from build123d import *

# Parameters (mm, degrees)
F1_DEPTH = 25
F2_R     = 1.5
F3_DEPTH = 25
F4_W     = 10
F4_H     = 10
F4_R     = 1.5
F5_DEPTH = 5
F6_SIZE  = 1
F7_SIZE  = 1


with BuildPart() as f1:
    # F0 (on Front) → F1 (new body)
    with BuildSketch(Plane.XZ):
        Polygon((0, -3.6), (0, 3.6), (10, 3.6), (10, 6.1), (-2.5, 6.1), (-2.5, -6.1), (15, -6.1), (15, -3.6), align=None)
    extrude(amount=F1_DEPTH)

    # F2 (on face) → F3 (cut)
    with BuildSketch(Plane.XY.offset(6.1)):
        with Locations((5.5, -5.5)):
            Circle(F2_R)
    extrude(amount=-F3_DEPTH, mode=Mode.SUBTRACT)

    # F4 (on face) → F5 (cut)
    with BuildSketch(Plane.XY.offset(6.1)):
        with Locations((5, -5)):
            Rectangle(F4_W, F4_H)
        with Locations((5.5, -5.5)):
            Circle(F4_R, mode=Mode.SUBTRACT)
    extrude(amount=-F5_DEPTH, mode=Mode.SUBTRACT)

    # F6
    f6_edges = [f1.edges().sort_by_distance(p)[0] for p in [
        (-2.5, -12.5, 6.1),
        (-2.5, -12.5, -6.1),
        (15, -12.5, -6.1),
        (6.25, -25, -6.1),
        (6.25, 0, -6.1),
        (-2.5, 0, 0),
    ]]
    chamfer(f6_edges, length=F6_SIZE)

    # F7
    f7_edges = [f1.edges().sort_by_distance(p)[0] for p in [
        (-0.75, 0, 6.1),
    ]]
    chamfer(f7_edges, length=F7_SIZE)


solid = f1.part
Check sheet for the modelled part. Datum: model origin and axes. Units: mm. A direction names the side the tool comes from. Coordinates: 2 decimals unless noted, no trailing zeros. Loops run counter-clockwise (first coordinate to the right, second up) from the corner with the lowest first, then second, coordinate; pieces in that order, holes last. Notation, with made-up numbers: (6.25, -30.5) -> (21.25, -30.5) arc R5 ccw to (21.25, -23.5) -> close; hole circle Ø9 at (49, 16.5). An arc over 180 degrees is marked (long way). Write item = value, one per line. Start each with the question number.
1. Section check D-D on z = -3. Record the cut outline in (x, y), then the cut area to 3 significant figures.
2. Material ranges on line 1 (Y direction, x = 5.5, z = -4.15); line 2 (Z direction, x = 1, y = -12.5); line 3 (X direction, y = -22.75, z = 0.75), recorded low to high.
3. Tool access check on faces 1 (the flat face through (10, -17, 5)), 2 (the flat face through (-2, -12.6, 5.6)), 3 (the flat face through (5, -10, 5)), 4 (the flat face through (5, -17, 3.6)). Record the directions out of +Z, -Z, +X, -X, +Y, -Y that give a thin tool (end or side, any length) a straight path to the whole face; none if there is none.
4. Draft check along Y on faces 5 (the flat face through (14.5, -12.3, -5.6)), 6 (the cylindrical face through (4.39, -4.49, -4.83)), 7 (the flat face through (-2, -0.5, 0.3)). Enter one of: released by +Y, released by -Y, zero draft, split by the parting line, or undercut.
5. Section check B-B on x = 5.5. Record the cut outline in (y, z), then the cut area to 3 significant figures.
6. Section check A-A on x = 8.25. Record the cut outline in (y, z), then the cut area to 3 significant figures.
7. Section check C-C on y = -5.5. Record the cut outline in (x, z).
8. Depth check by flat-ended pin: P1, Ø5, axis at x = 5.5, y = -5.5, coming from the +Z side; P2, Ø2, axis at x = 6, z = 5, coming from the +Y side; P3, Ø1.2, axis at y = -20, z = 5.5, coming from the +X side. Enter the tip coordinate at first touch or a pass-through.
Responses:
q1.outline = (-2.5, -25) -> (0, -25) -> (0, 0) -> (-1.5, 0) -> (-2.5, -1) -> close
q1.area = 62.0 mm2
q2.line_1 = -25 to -7, -4 to 0
q2.line_2 = -6.1 to -3.6, 3.6 to 6.1
q2.line_3 = -2.5 to 0
q3.face_1 = +Z, +X, +Y, -Y
q3.face_2 = +Z, -X, +Y, -Y
q3.face_3 = +Z, +X, +Y
q3.face_4 = +X, +Y, -Y
q4.face_5 = zero draft
q4.face_6 = undercut
q4.face_7 = released by +Y
q5.outline = (-25, -5.1) -> (-24, -6.1) -> (-7, -6.1) -> (-7, -3.6) -> (-25, -3.6) -> close; (-25, 3.6) -> (-10, 3.6) -> (-10, 6.1) -> (-25, 6.1) -> close; (-4, -6.1) -> (-1, -6.1) -> (0, -5.1) -> (0, -3.6) -> (-4, -3.6) -> close
q5.area = 91.5 mm2
q6.outline = (-25, -5.1) -> (-24, -6.1) -> (-1, -6.1) -> (0, -5.1) -> (0, -3.6) -> (-25, -3.6) -> close; (-25, 3.6) -> (-10, 3.6) -> (-10, 6.1) -> (-25, 6.1) -> close
q6.area = 99.0 mm2
q7.outline = (-2.5, -5.1) -> (-1.5, -6.1) -> (4, -6.1) -> (4, -3.6) -> (0, -3.6) -> (0, 6.1) -> (-1.5, 6.1) -> (-2.5, 5.1) -> close; (7, -6.1) -> (14, -6.1) -> (15, -5.1) -> (15, -3.6) -> (7, -3.6) -> close
q8.P1 = -3.6
q8.P2 = -10
q8.P3 = 10
